from build123d import *

# Parameters (mm, degrees)
BOSS_EXTRUDE2_DEPTH = 35
BOSS_EXTRUDE3_DEPTH = 5
SCALE1_SCALE        = 0.3


with BuildPart() as part:
    # Sketch2 → Boss-Extrude2 (new body)
    with BuildSketch(Plane(origin=(0, 0, 0), x_dir=(1, 0, 0), z_dir=(0, 1, 0))):
        with BuildLine():
            Line((-10, 107.320508076), (-87.942286341, 62.320508076))
            ThreePointArc((-87.942286341, 62.320508076), (-95.262794416, 55), (-97.942286341, 45))
            Line((-97.942286341, 45), (-97.942286341, -45))
            ThreePointArc((-97.942286341, -45), (-95.262794416, -55), (-87.942286341, -62.320508076))
            Line((-87.942286341, -62.320508076), (-10, -107.320508076))
            ThreePointArc((-10, -107.320508076), (0, -110), (10, -107.320508076))
            Line((10, -107.320508076), (87.942286341, -62.320508076))
            ThreePointArc((87.942286341, -62.320508076), (95.262794416, -55), (97.942286341, -45))
            Line((97.942286341, -45), (97.942286341, 45))
            ThreePointArc((97.942286341, 45), (95.262794416, 55), (87.942286341, 62.320508076))
            Line((87.942286341, 62.320508076), (10, 107.320508076))
            ThreePointArc((10, 107.320508076), (0, 110), (-10, 107.320508076))
        make_face()
    extrude(amount=BOSS_EXTRUDE2_DEPTH)

    # Sketch5 → Boss-Extrude3 (add)
    with BuildSketch(Plane(origin=(0, 35, 0), x_dir=(1, 0, 0), z_dir=(0, 1, 0))):
        with BuildLine():
            Line((-10, 112.320508076), (-92.27241336, 64.820508076))
            ThreePointArc((-92.27241336, 64.820508076), (-99.592921435, 57.5), (-102.27241336, 47.5))
            Line((-102.27241336, 47.5), (-102.27241336, -47.5))
            ThreePointArc((-102.27241336, -47.5), (-99.592921435, -57.5), (-92.27241336, -64.820508076))
            Line((-92.27241336, -64.820508076), (-10, -112.320508076))
            ThreePointArc((-10, -112.320508076), (0, -115), (10, -112.320508076))
            Line((10, -112.320508076), (92.27241336, -64.820508076))
            ThreePointArc((92.27241336, -64.820508076), (99.592921435, -57.5), (102.27241336, -47.5))
            Line((102.27241336, -47.5), (102.27241336, 47.5))
            ThreePointArc((102.27241336, 47.5), (99.592921435, 57.5), (92.27241336, 64.820508076))
            Line((92.27241336, 64.820508076), (10, 112.320508076))
            ThreePointArc((10, 112.320508076), (0, 115), (-10, 112.320508076))
        make_face()
    extrude(amount=BOSS_EXTRUDE3_DEPTH)


with BuildPart() as part_1:
    # Scale1: scaled about (0, 20.196243732, 0)
    add(part.part.scale(SCALE1_SCALE).moved(Location((0, 14.137370612, 0))))


solid = part_1.part
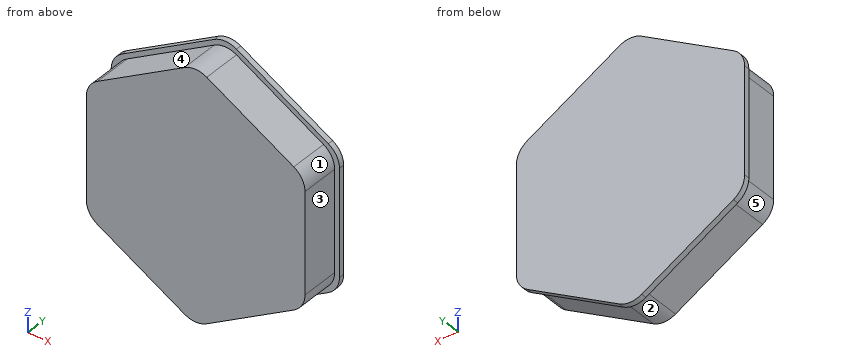
Verification items for the finished model (mm, model axes). Face numbers are marked on the shaded views. A direction names the side the tool comes from. Give positions to 0.01 mm unless a question says otherwise; leave off trailing zeros. Loops run counter-clockwise (first coordinate to the right, second up) from the corner with the lowest first, then second, coordinate; pieces in that order, holes last.
1. Go/stop test with flat-tipped pins: P1, Ø2, axis at x = 9.5, y = 21, coming from the +Z side; P2, Ø3, axis at y = 19.5, z = 5.5, coming from the -X side; P3, Ø1.5, axis at x = 2.5, y = 21, coming from the -Z side. Record where each tip stops, or that it passes through.
Derived:
P1: stops at z = 29.02
P2: stops at x = -29.38
P3: stops at z = -32.74
2. Cross-section at A-A on y = 15.25. Record the cut outline in (x, z), and give its area (3 significant figures).
Derived:
outline: (-29.38, -13.5) arc R6 ccw to (-26.38, -18.7) - (-3, -32.2) arc R6 ccw to (3, -32.2) - (26.38, -18.7) arc R6 ccw to (29.38, -13.5) - (29.38, 13.5) arc R6 ccw to (26.38, 18.7) - (3, 32.2) arc R6 ccw to (-3, 32.2) - (-26.38, 18.7) arc R6 ccw to (-29.38, 13.5) - close
area: 2,980 mm2
3. Cross-section at B-B on z = -12.5. Record the cut outline in (x, y), and give its area (3 significant figures).
Derived:
outline: (-30.68, 24.64) - (-29.38, 24.64) - (-29.38, 14.14) - (29.38, 14.14) - (29.38, 24.64) - (30.68, 24.64) - (30.68, 26.14) - (-30.68, 26.14) - close
area: 709 mm2
4. Tool access check on the marked faces 1, 2, 3, 4 and 5. Record the directions out of +Z, -Z, +X, -X, +Y, -Y that give a thin tool (end or side, any length) a straight path to the whole face; none if there is none.
Derived:
face 1: +Z, +X, -Y
face 2: -Z, -Y
face 3: +Z, -Z, +X, -Y
face 4: +Z, -X, -Y
face 5: -Z, -X, -Y
5. Material ranges on probe 1 along X at (y, z) = (20.75, 5); probe 2 along Z at (x, y) = (-16, 22.5); probe 3 along X at (y, z) = (24, 19), recorded low to high.
Derived:
probe 1: x = -29.38 to 29.38
probe 2: z = -24.69 to 24.69
probe 3: x = -25.86 to 25.86
6. Cross-section at C-C on x = 12. Record the cut outline in (y, z).
Derived:
outline: (14.14, -27) - (24.64, -27) - (24.64, -28.5) - (26.14, -28.5) - (26.14, 28.5) - (24.64, 28.5) - (24.64, 27) - (14.14, 27) - close
